Could you check a few things on this model? Use its own coordinates, in mm. A direction names the side the tool comes from. Give positions to 0.01 mm unless a question says otherwise; leave off trailing zeros. Loops run counter-clockwise (first coordinate to the right, second up) from the corner with the lowest first, then second, coordinate; pieces in that order, holes last. Notation, with made-up numbers: (61, 15) -> (96, 15) arc R19 cw to (96, 37) -> close; hole circle Ø3 at (-26.75, -25.5). An arc over 180 degrees is marked (long way). Write item = value, one per line. Start each with the question number.
1) I want a section at A-A (z = 30.85). List the corners of the cut face in (x, y) for me.
2) I need wall thicknesses on probe 1 along X at (y, z) = (1.3, 10); probe 2 along X at (y, z) = (1.4, -10); probe 3 along Z at (x, y) = (-6, 1.3). Which ranges of each line are inside material? Lowest first, please. Write a range as from..to.
3) I'm going to push flat-ended pins straight in: pin 1 Ø2 at (x, z) = (7.5, 10) entering from +Y; pin 2 Ø4 at (x, z) = (-30.85, -55.65) entering from -Y; pin 3 Ø1.5 at (x, z) = (8.5, -9.5) entering from +Y; pin 4 Ø1 at (x, y) = (-32, 1) entering from +Z. Where does each tip first touch, or does it pass through?
4) I want a section at D-D (x = 30.85). List the corners of the cut face in (y, z) for me, and give its area (3 significant figures).
5) If we mould it in two halves opening along X, with no side actions, what happens to faces 6 (the face through (41.152, 0.986, 17.096)), 7 (the face through (5.06, 1.51, -10.54)), 8 (the face through (-6.944, 1.014, -26.12)), 9 (the face through (-4, 0, -5))? For each: +X half, -X half, draft (parallel to the pull), parting line (faces both ways), or undercut.
6) I want a section at B-B (z = -49). List the corners of the cut face in (x, y) for me, and give its area (3 significant figures).
7) I want a section at C-C (y = 0.55). Count the separate pieces of the cut face and the enclosed holes in it, and give its area (3 significant figures).
8) On a 3-axis mill with a long thin cutter (end or side, diameter ignored), from which of +Z, -Z, +X, -X, +Y, -Y can I reach the whole of each face in a straight line? I mean faces 1 (the face through (-26.12, 1.014, 6.944)), 2 (the face through (5.06, 1.51, 9.46)), 3 (the face through (54.385, 0.986, 30.044)), 4 (the face through (-18.848, 0.986, -44.313)), 5 (the face through (-39.46, 0.99, 27.59)). Say none if no direction works.
from build123d import *

# Parameters (mm, degrees)
SKETCH1_R           = 25
SKETCH1_R_2         = 1.1
BOSS_EXTRUDE1_DEPTH = 2
SKETCH2_R           = 2.5
CUT_EXTRUDE1_DEPTH  = 1
SKETCH3_R           = 1.5
BOSS_EXTRUDE2_DEPTH = 2
FILLET1_R           = 10
FILLET2_R           = 10


with BuildPart() as part:
    # Sketch1 → Boss-Extrude1 (new body)
    with BuildSketch(Plane(origin=(0, 0, 0), x_dir=(1, 0, 0), z_dir=(0, 1, 0))):
        with Locations(Location((0, 0, 0), (0, 0, 270))):
            Circle(SKETCH1_R)
        with Locations(Location((-7.5, 10, 0), (0, 0, 270))):
            Circle(SKETCH1_R_2, mode=Mode.SUBTRACT)
        with Locations(Location((7.5, 10, 0), (0, 0, 270))):
            Circle(SKETCH1_R_2, mode=Mode.SUBTRACT)
        with Locations(Location((-7.5, -10, 0), (0, 0, 270))):
            Circle(SKETCH1_R_2, mode=Mode.SUBTRACT)
        with Locations(Location((7.5, -10, 0), (0, 0, 270))):
            Circle(SKETCH1_R_2, mode=Mode.SUBTRACT)
    extrude(amount=BOSS_EXTRUDE1_DEPTH)

    # Sketch2 → Cut-Extrude1 (cut)
    with BuildSketch(Plane(origin=(0, 2, 0), x_dir=(1, 0, 0), z_dir=(0, 1, 0))):
        with Locations(Location((-7.5, 10, 0), (0, 0, 270))):
            Circle(SKETCH2_R)
        with Locations(Location((7.5, 10, 0), (0, 0, 270))):
            Circle(SKETCH2_R)
        with Locations(Location((-7.5, -10, 0), (0, 0, 270))):
            Circle(SKETCH2_R)
        with Locations(Location((7.5, -10, 0), (0, 0, 270))):
            Circle(SKETCH2_R)
    extrude(amount=-CUT_EXTRUDE1_DEPTH, mode=Mode.SUBTRACT)

    # Sketch3 → Boss-Extrude2 (add)
    # profile 1 of 4: a face of its own
    with BuildSketch(Plane(origin=(0, 0, 0), x_dir=(1, 0, 0), z_dir=(0, 1, 0))):
        with BuildLine():
            Line((-7.503148867, 23.847489534), (-26.96183357, 58.948812182))
            ThreePointArc((-26.96183357, 58.948812182), (-29.357833738, 60.85453152), (-32.399608771, 60.507850621))
            Line((-32.399608771, 60.507850621), (-34.148812182, 59.53816643))
            ThreePointArc((-34.148812182, 59.53816643), (-36.05453152, 57.142166262), (-35.707850621, 54.100391229))
            Line((-35.707850621, 54.100391229), (-16.249165919, 18.999068581))
            ThreePointArc((-16.249165919, 18.999068581), (-12.121052382, 21.865042628), (-7.503148867, 23.847489534))
        make_face()
        with Locations(Location((-30.85, 55.65, 0), (0, 0, 270))):
            Circle(SKETCH3_R, mode=Mode.SUBTRACT)
    # profile 2 of 4: a face of its own
    with BuildSketch(Plane(origin=(0, 0, 0), x_dir=(1, 0, 0), z_dir=(0, 1, 0))):
        with BuildLine():
            Line((-58.948812182, -26.96183357), (-23.847489534, -7.503148867))
            ThreePointArc((-23.847489534, -7.503148867), (-21.865042628, -12.121052382), (-18.999068581, -16.249165919))
            Line((-18.999068581, -16.249165919), (-54.100391229, -35.707850621))
            ThreePointArc((-54.100391229, -35.707850621), (-57.142166262, -36.05453152), (-59.53816643, -34.148812182))
            Line((-59.53816643, -34.148812182), (-60.507850621, -32.399608771))
            ThreePointArc((-60.507850621, -32.399608771), (-60.85453152, -29.357833738), (-58.948812182, -26.96183357))
        make_face()
        with Locations(Location((-55.65, -30.85, 0), (0, 0, 270))):
            Circle(SKETCH3_R, mode=Mode.SUBTRACT)
    # profile 3 of 4: a face of its own
    with BuildSketch(Plane(origin=(0, 0, 0), x_dir=(1, 0, 0), z_dir=(0, 1, 0))):
        with BuildLine():
            Line((60.507850621, -32.399608771), (59.53816643, -34.148812182))
            ThreePointArc((59.53816643, -34.148812182), (57.142166262, -36.05453152), (54.100391229, -35.707850621))
            Line((54.100391229, -35.707850621), (18.999068581, -16.249165919))
            ThreePointArc((18.999068581, -16.249165919), (21.865042628, -12.121052382), (23.847489534, -7.503148867))
            Line((23.847489534, -7.503148867), (58.948812182, -26.96183357))
            ThreePointArc((58.948812182, -26.96183357), (60.85453152, -29.357833738), (60.507850621, -32.399608771))
        make_face()
        with Locations(Location((55.65, -30.85, 0), (0, 0, 90))):
            Circle(SKETCH3_R, mode=Mode.SUBTRACT)
    # profile 4 of 4: a face of its own
    with BuildSketch(Plane(origin=(0, 0, 0), x_dir=(1, 0, 0), z_dir=(0, 1, 0))):
        with BuildLine():
            Line((32.399608771, 60.507850621), (34.148812182, 59.53816643))
            ThreePointArc((34.148812182, 59.53816643), (36.05453152, 57.142166262), (35.707850621, 54.100391229))
            Line((35.707850621, 54.100391229), (16.249165919, 18.999068581))
            ThreePointArc((16.249165919, 18.999068581), (12.121052382, 21.865042628), (7.503148867, 23.847489534))
            Line((7.503148867, 23.847489534), (26.96183357, 58.948812182))
            ThreePointArc((26.96183357, 58.948812182), (29.357833738, 60.85453152), (32.399608771, 60.507850621))
        make_face()
        with Locations(Location((30.85, 55.65, 0), (0, 0, 90))):
            Circle(SKETCH3_R, mode=Mode.SUBTRACT)
    extrude(amount=BOSS_EXTRUDE2_DEPTH)

    # Fillet1
    fillet1_edges = [part.edges().sort_by_distance(p)[0] for p in [
        (-7.503148867, 1, -23.847489534),
        (-16.249165919, 1, -18.999068581),
        (-23.847489534, 1, 7.503148867),
        (-18.999068581, 1, 16.249165919),
        (18.999068581, 1, 16.249165919),
        (16.249165919, 1, -18.999068581),
    ]]
    fillet(fillet1_edges, radius=FILLET1_R)

    # Fillet2
    fillet2_edges = [part.edges().sort_by_distance(p)[0] for p in [
        (7.503148867, 1, -23.847489534),
    ]]
    fillet(fillet2_edges, radius=FILLET2_R)


solid = part.part
Answer list:
q1.outline = (-60.99, 0) -> (-57.15, 0) -> (-57.15, 2) -> (-60.99, 2) -> close; (-54.15, 0) -> (-45.34, 0) -> (-45.34, 2) -> (-54.15, 2) -> close; (45.34, 0) -> (54.15, 0) -> (54.15, 2) -> (45.34, 2) -> close; (57.15, 0) -> (60.99, 0) -> (60.99, 2) -> (57.15, 2) -> close
q2.probe_1 = -28.66..-10, -5..5, 10..28.35
q2.probe_2 = -22.91..-10, -5..5, 10..22.91
q2.probe_3 = -25.67..-12, -8..8, 12..24.27
q3.pin_1 = through
q3.pin_2 = 0
q3.pin_3 = 1
q3.pin_4 = 23.73
q4.outline = (0, -60.99) -> (2, -60.99) -> (2, -57.15) -> (0, -57.15) -> close; (0, -54.15) -> (2, -54.15) -> (2, -45.34) -> (0, -45.34) -> close; (0, 11.39) -> (2, 11.39) -> (2, 22.82) -> (0, 22.82) -> close
q4.area = 48.2 mm^2
q5.face_6 = +X half
q5.face_7 = undercut
q5.face_8 = undercut
q5.face_9 = draft
q6.outline = (-32.88, 0) -> (-21.45, 0) -> (-21.45, 2) -> (-32.88, 2) -> close; (21.45, 0) -> (32.88, 0) -> (32.88, 2) -> (21.45, 2) -> close
q6.area = 45.7 mm^2
q7.separate_pieces = 1
q7.enclosed_holes = 8
q7.area = 3,700 mm^2
q8.face_1 = -X, +Y, -Y
q8.face_2 = +Y
q8.face_3 = +Y, -Y
q8.face_4 = -Z, +Y, -Y
q8.face_5 = +Z, +Y, -Y
